Verification items for the finished model (mm, model axes). Round coordinates to 2 decimals unless told otherwise and drop trailing zeros. Write each loop counter-clockwise with the first axis right and the second up, starting at its lowest first coordinate (ties: lowest second). Pieces come first, ordered by that corner, then holes. Notation, with made-up numbers: M 68,-35 L 87,-35 A9 ccw 87,-25 Z; hole C 70,31 d11. An arc over 180 degrees is marked long. One line per question, with ' | ' between items. Start each with the question number.
Q1. Gauge pin test, flat ends, axial feed: pin 1 (5 mm diameter, centred on x = 5.5, y = 36.58, fed in from +Z); pin 2 (2.5 mm diameter, centred on x = 10.5, y = 76, fed in from +Z). Record the tip position at first contact, or that the pin passes through.
Q2. Cross-section at B-B (y = 5.58). Record the boundary of the cut face in (x, z) (3 decimals), then the cut area to 3 significant figures.
Q3. Cross-section at C-C (x = 31). Record the boundary of the cut face in (y, z), then the cut area to 3 significant figures.
Q4. Cross-section at D-D (y = 21.08). Record the boundary of the cut face in (x, z).
Q5. Thickness scan on line 1 along Y through (x, z) = (11, 3.55); line 2 along X through (y, z) = (56.8, 1.15); line 3 along Y through (x, z) = (31, 0.85). Record the ranges inside material, lowest first. Write a range as from..to.
Q6. Cross-section at A-A (x = 21). Record the boundary of the cut face in (y, z), then the cut area to 3 significant figures.
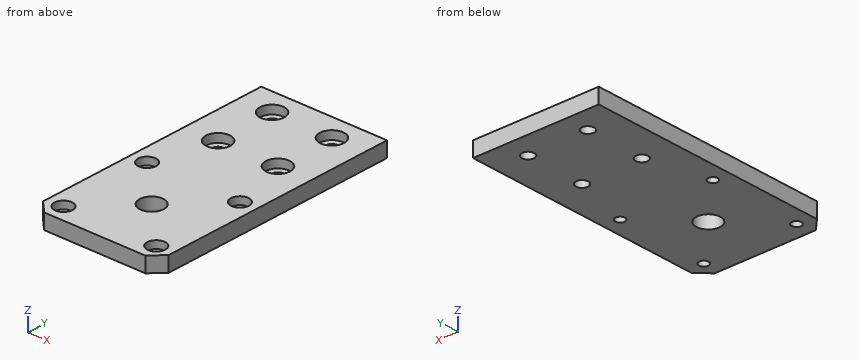
from build123d import *

# Parameters (mm, degrees)
CROQUIS1_W              = 42
CROQUIS1_H              = 85
CROQUIS1_R              = 2.05
SALIENTE_EXTRUIR1_DEPTH = 5
CROQUIS4_R              = 4.05
CORTAR_EXTRUIR1_DEPTH   = 2.8
CROQUIS5_R              = 1.575
CROQUIS5_R_2            = 4
CORTAR_EXTRUIR2_DEPTH   = 6
CROQUIS6_R              = 3
CORTAR_EXTRUIR3_DEPTH   = 2.5
CHAFL_N1_SIZE           = 4.1


with BuildPart() as part:
    # Croquis1 → Saliente-Extruir1 (new body)
    with BuildSketch(Plane.XY):
        with Locations((21, 42.5)):
            Rectangle(CROQUIS1_W, CROQUIS1_H)
        with Locations((11, 76.8)):
            Circle(CROQUIS1_R, mode=Mode.SUBTRACT)
        with Locations((31, 76.8)):
            Circle(CROQUIS1_R, mode=Mode.SUBTRACT)
        with Locations((31, 56.8)):
            Circle(CROQUIS1_R, mode=Mode.SUBTRACT)
        with Locations((11, 56.8)):
            Circle(CROQUIS1_R, mode=Mode.SUBTRACT)
    extrude(amount=SALIENTE_EXTRUIR1_DEPTH)

    # Croquis4 → Cortar-Extruir1 (cut)
    with BuildSketch(Plane.XY.offset(5)):
        with Locations((11, 76.8)):
            Circle(CROQUIS4_R)
        with Locations((11, 56.8)):
            Circle(CROQUIS4_R)
        with Locations((31, 56.8)):
            Circle(CROQUIS4_R)
        with Locations((31, 76.8)):
            Circle(CROQUIS4_R)
    extrude(amount=-CORTAR_EXTRUIR1_DEPTH, mode=Mode.SUBTRACT)

    # Croquis5 → Cortar-Extruir2 (cut, through all)
    with BuildSketch(Plane.XY.offset(5)):
        with Locations((5.5, 36.58)):
            Circle(CROQUIS5_R)
        with Locations((36.5, 36.58)):
            Circle(CROQUIS5_R)
        with Locations((36.5, 5.58)):
            Circle(CROQUIS5_R)
        with Locations((5.5, 5.58)):
            Circle(CROQUIS5_R)
        with Locations((21, 21.08)):
            Circle(CROQUIS5_R_2)
    extrude(amount=-CORTAR_EXTRUIR2_DEPTH, mode=Mode.SUBTRACT)

    # Croquis6 → Cortar-Extruir3 (cut)
    with BuildSketch(Plane.XY.offset(5)):
        with Locations((5.5, 36.58)):
            Circle(CROQUIS6_R)
        with Locations((36.5, 36.58)):
            Circle(CROQUIS6_R)
        with Locations((36.5, 5.58)):
            Circle(CROQUIS6_R)
        with Locations((5.5, 5.58)):
            Circle(CROQUIS6_R)
    extrude(amount=-CORTAR_EXTRUIR3_DEPTH, mode=Mode.SUBTRACT)

    # Chaflán1
    chafl_n1_edges = [part.edges().sort_by_distance(p)[0] for p in [
        (42, 0, 2.5),
        (0, 0, 2.5),
    ]]
    chamfer(chafl_n1_edges, length=CHAFL_N1_SIZE)


solid = part.part
Determined:
1) pin 1: stops at z = 2.5 | pin 2: stops at z = 2.2
2) outline: M 0,0 L 3.925,0 L 3.925,2.5 L 2.5,2.5 L 2.5,5 L 0,5 Z; M 7.075,0 L 34.925,0 L 34.925,2.5 L 33.5,2.5 L 33.5,5 L 8.5,5 L 8.5,2.5 L 7.075,2.5 Z; M 38.075,0 L 42,0 L 42,5 L 39.5,5 L 39.5,2.5 L 38.075,2.5 Z | area: 164 mm²
3) outline: M 0,0 L 54.75,0 L 54.75,2.2 L 52.75,2.2 L 52.75,5 L 0,5 Z; M 58.85,0 L 74.75,0 L 74.75,2.2 L 72.75,2.2 L 72.75,5 L 60.85,5 L 60.85,2.2 L 58.85,2.2 Z; M 78.85,0 L 85,0 L 85,5 L 80.85,5 L 80.85,2.2 L 78.85,2.2 Z | area: 362 mm²
4) outline: M 0,0 L 17,0 L 17,5 L 0,5 Z; M 25,0 L 42,0 L 42,5 L 25,5 Z
5) line 1: y = 0..52.75, 60.85..72.75, 80.85..85 | line 2: x = 0..8.95, 13.05..28.95, 33.05..42 | line 3: y = 0..54.75, 58.85..74.75, 78.85..85
6) outline: M 0,0 L 17.08,0 L 17.08,5 L 0,5 Z; M 25.08,0 L 85,0 L 85,5 L 25.08,5 Z | area: 385 mm²
